from build123d import *

# Parameters (mm, degrees)
F0_W     = 128.64919
F0_H     = 107.927158
F1_DEPTH = 25.4
F3_R     = 29.576155
F4_DEPTH = 36.322
F6_DEPTH = 38.1
F7_DEPTH = 62.992


with BuildPart() as f1:
    # F0 (on Top) → F1 (new body)
    with BuildSketch(Plane.XY):
        Rectangle(F0_W, F0_H)
    extrude(amount=F1_DEPTH)

    # F3 (on face) → F4 (join)
    with BuildSketch(Plane.XY.offset(25.4)):
        Circle(F3_R)
    extrude(amount=F4_DEPTH)

    # F5 (on Front) → F6 (cut)
    with BuildSketch(Plane.XZ):
        Polygon((-54.256331, 60.477722), (-46.154052, 55.84785), (49.91582, 41.379493), (30.238859, 72.631143), align=None)
    extrude(amount=-F6_DEPTH, mode=Mode.SUBTRACT)

    # F5 (on Front) → F7 (cut)
    with BuildSketch(Plane.XZ):
        Polygon((-54.256331, 60.477722), (-46.154052, 55.84785), (49.91582, 41.379493), (30.238859, 72.631143), align=None)
    extrude(amount=F7_DEPTH, mode=Mode.SUBTRACT)


solid = f1.part
Verification items for the finished model (mm, model axes). A direction names the side the tool comes from. Coordinates: 2 decimals unless noted, no trailing zeros. Order: outer loops, then holes, each group sorted by start corner. A loop starts at its lowest first (then second) coordinate and runs counter-clockwise, first axis right, second up.
1. Sectioned sample at D-D, the plane y = 47. Record the cut outline in (x, z), and give its area (3 significant figures).
Results found:
outline: (-64.32, 0) - (64.32, 0) - (64.32, 25.4) - (-64.32, 25.4) - close
area: 3,270 mm2
2. Set-up check for faces 1 (the face through (64.325, -1, 13)), 2 (the face through (-29.548, 1.3, 36.074)): record each of +Z, -Z, +X, -X, +Y, -Y from which the full face is reachable in a straight line by a thin tool's end or side.
Results found:
face 1: +Z, -Z, +X, +Y, -Y
face 2: +Z
3. Sectioned sample at C-C, the plane z = 34.5. Record the cut outline in (x, y).
Results found:
outline: circle Ø59.15 at (0, 0)
4. Scan lines: line 1 (Y direction, x = 1, z = 38.5); line 2 (Z direction, x = 37, y = -38); line 3 (Y direction, x = 18, z = 31.5). Record each from-to range of solid material in increasing order.
Results found:
line 1: y = -29.56 to 29.56
line 2: z = 0 to 25.4
line 3: y = -23.47 to 23.47
5. Sectioned sample at B-B, the plane x = 0. Record the cut outline in (y, z).
Results found:
outline: (-53.96, 0) - (53.96, 0) - (53.96, 25.4) - (29.58, 25.4) - (29.58, 48.9) - (-29.58, 48.9) - (-29.58, 25.4) - (-53.96, 25.4) - close
6. Go/stop test with a flat-tipped pin: pin 1 Ø6 at (x, z) = (-4, 43) entering from -Y. Record where the tip stops, or that it passes through.
Results found:
pin 1: stops at y = -29.56
7. Sectioned sample at A-A, the plane y = 0. Record the cut outline in (x, z).
Results found:
outline: (-64.32, 0) - (64.32, 0) - (64.32, 25.4) - (29.58, 25.4) - (29.58, 44.44) - (-29.58, 53.35) - (-29.58, 25.4) - (-64.32, 25.4) - close
